CAD build for the part. Positions are in the model's coordinates, mm. A direction names the side the tool comes from. Coordinates: 2 decimals unless noted, no trailing zeros. Loops run counter-clockwise (first coordinate to the right, second up) from the corner with the lowest first, then second, coordinate; pieces in that order, holes last. Notation, with made-up numbers: (24.25, -16.75) -> (69.25, -16.75) arc R11 cw to (69.25, -4.75) -> close; hole circle Ø11 at (82.25, 87). An arc over 180 degrees is marked (long way). Write each question's results on one line, items separated by ' | '.
Autodesk Inventor part; units mm, degrees
ref_plane "YZ Plane" through (0, 0, 0) normal (1, 0, 0) x (0, 1, 0)
ref_plane "XZ Plane" through (0, 0, 0) normal (0, 1, 0) x (-1, 0, 0)
ref_plane "XY Plane" through (0, 0, 0) normal (0, 0, 1) x (1, 0, 0)
sketch "スケッチ1" plane through (0, 0, 0) normal (0, 1, 0) x (-1, 0, 0)
  line L0 (0, 0) -> (20, 0)
  line L1 (20, 0) -> (20, -40)
  line L2 (20, -40) -> (0, -40)
  line L3 (0, -40) -> (0, 0)
  circle A0 centre (0, -20) radius 13.6
  circle A1 centre (0, -20) radius 17.5
  line L4 (0, -6.4) -> (4, -6.4)
  line L5 (4, -6.4) -> (4, 3.6)
  line L6 (4, 3.6) -> (0, 3.6)
  line L7 (0, 3.6) -> (0, -6.4)
  line L8 (0, -33.6) -> (4, -33.6)
  line L9 (4, -33.6) -> (4, -43.6)
  line L10 (4, -43.6) -> (0, -43.6)
  line L11 (0, -43.6) -> (0, -33.6)
  point P0 (0, -6.4)
  point P1 (0, -33.6)
  point P2 (4, -37.0367)
  point P3 (4, -2.9633)
  dimension "d0" = 20
  dimension "d1" = 40
  dimension "d2" = 27.2
  dimension "d3" = 35
  dimension "d4" = 4
  dimension "d5" = 10
  dimension "d6" = 4
  dimension "d7" = 10
extrude "押し出し1" add sketch "スケッチ1" along normal blind 87 contours L7 L6 L5 L0 | L0 L5 A1 L3 | A1 L5 L4 L3 | A1 L9 L8 A0 L4 L5 | A1 L9 L2 L3 | L3 L8 L9 A1 | L2 L9 L10 L11
sketch "スケッチ2" plane through (-4, 0, -43.6) normal (-1, 0, 0) x (0, 0, 1)
  line L0 (0, 87) -> (6.5633, 87)
  line L1 (40.6367, 87) -> (47.2, 87)
  line L2 (40.6367, 0) -> (47.2, 0)
  line L3 (0, 0) -> (6.5633, 0)
  point P0 (43.6, 0)
  point P1 (3.2816, 13)
  point P2 (3.2816, 79)
  point P3 (43.9184, 79)
  point P4 (43.9184, 13)
  point P5 (3.2816, 87)
  point P6 (43.9184, 87)
  point P7 (43.9184, 0)
  point P8 (3.2816, 0)
  dimension "d10" = 0
  dimension "d11" = 8
  dimension "d12" = 0
  dimension "d13" = 8
  dimension "d14" = 0
  dimension "d15" = 0
  dimension "d16" = 13
  dimension "d17" = 13
hole "穴1" at (-4, 13, -40.3184) at (-4, 79, -40.3184) at (-4, 79, 0.3184) at (-4, 13, 0.3184) direction (1, 0, 0) diameter 3 end through all
fillet "フィレット1" radius 1 14 edges at (-4, 87, 0.3184) (-17.5, 87, -20) (-4, 87, -40.3184) (-2, 87, -43.6) (-2, 87, 3.6) (-4, 43.5, 3.6) (-4, 0, 0.3184) (-17.5, 0, -20) (-4, 0, -40.3184) (-2, 0, -43.6) (-2, 0, 3.6) (-4, 43.5, -43.6) (-4, 43.5, -37.0367) (-4, 43.5, -2.9633)
sketch "スケッチ3" plane through (0, 87, 0) normal (0, 1, 0) x (1, 0, 0)
  line L0 (0, -2.6) -> (-3, -2.6)
  line L1 (-3, 42.6) -> (0, 42.6)
  circle A0 centre (-1.5, 39.6) radius 0.5
  circle A1 centre (-1.5, 0.4) radius 0.5
  circle A2 centre (-15.1647, 20) radius 0.5
  arc A3 (-4.7297, 36.8487) -> (-4.7297, 3.1513) centre (0, 20) ccw
  point P0 (-17.5, 20)
  dimension "d28" = 3
  dimension "d29" = 3
  dimension "d30" = 1
  dimension "d31" = 1
  dimension "d32" = 1
  dimension "d33" = 0
extrude "押し出し2" add sketch "スケッチ3" along normal blind 2
sketch "スケッチ4" plane through (-1.5, 89, -39.6) normal (0, 1, 0) x (1, 0, 0)
  line L0 (-16.7138, 4.8708) -> (4.6687, 4.8708)
  line L1 (4.6687, 4.8708) -> (4.6687, -44.2225)
  line L2 (4.6687, -44.2225) -> (-16.7138, -44.2225)
  line L3 (-16.7138, -44.2225) -> (-16.7138, 4.8708)
  point P0 (1.5, -39.6)
extrude "押し出し3" add sketch "スケッチ4" along normal blind 1
sketch "スケッチ5" plane through (-4, 1, -37.8115) normal (-1, 0, 0) x (0, 0, 1)
  circle A0 centre (-2.5068, 12) radius 1.5
  circle A1 centre (-2.5068, 12) radius 2.5
  circle A2 centre (38.1299, 12) radius 1.5
  circle A3 centre (38.1299, 12) radius 2.5
  circle A4 centre (-2.5068, 78) radius 1.5
  circle A5 centre (-2.5068, 78) radius 2.5
  circle A6 centre (38.1299, 78) radius 1.5
  circle A7 centre (38.1299, 78) radius 2.5
  point P0 (37.8115, -1)
  dimension "d36" = 5
  dimension "d37" = 5
  dimension "d38" = 5
  dimension "d39" = 5
extrude "押し出し4" cut sketch "スケッチ5" against normal blind 2
properties part number "arm-2-2_3D プリント"
Q1. Cut at B-B on y = 13. Give the number of separate pieces and of enclosed holes in the cut face, and give its area (3 significant figures).
Results are:
separate pieces: 3 | enclosed holes: 0 | area: 208 mm^2
Q2. Wall check: L1, parallel to Z at x = -0.5, y = 79; L2, parallel to Z at x = -3.1, y = 79; L3, parallel to Y at x = -2, z = -35. Give the ranges that are in metal, low to high. Write a range as from..to.
Results are:
L1: -43.6..-41.82, -38.82..-33.59, -6.41..-1.18, 1.82..3.6 | L2: -43.59..-42.82, -37.82..-33.24, -6.76..-2.18, 2.82..3.59 | L3: 0..87, 89..90
Q3. Pull direction Z, two halves, no side cores. Call faces 5 (the flat face through (0, 43, -1)), 6 (the cylindrical face through (-3.01, 10.56, -0.22)), 7 (the cylindrical face through (-0.986, 77.735, 1.125)), 8 (the cylindrical face through (-17.497, 42.905, -19.682)): +Z half, -Z half, draft (parallel to the pull), parting line (faces both ways), or undercut.
Results are:
face 5: draft | face 6: undercut | face 7: undercut | face 8: parting line
Q4. Which spindle directions (+Z, -Z, +X, -X, +Y, -Y) get a long thin tool onto all of the face, cutting with end or side? Do faces 1 (the flat face through (-4, 43, 0)), 2 (the cylindrical face through (-3.01, 78.04, -38.01)), 3 (the cylindrical face through (-13.597, 42.891, -19.701)), 4 (the flat face through (-2, 43, 3.6)). Say none if no direction does.
Results are:
face 1: +Z, -X, -Y | face 2: -X | face 3: +X, -Y | face 4: +Z, +X, -X, -Y
Q5. Cut at D-D on x = 1.5. Write the cut outline in (y, z), and give its area (3 significant figures).
Results are:
outline: (89, -44.47) -> (90, -44.47) -> (90, 4.62) -> (89, 4.62) -> close | area: 49.1 mm^2
Q6. Drop flat-ended pins along their axis: pin 1 (6 mm diameter, centred on y = 29, z = -9, fed in from -X); pin 2 (1.5 mm diameter, centred on x = -1, y = 25, fed in from -Z); pin 3 (4 mm diameter, centred on x = -7, y = 16.5, fed in from -Z); pin 4 (1.8 mm diameter, centred on y = 13, z = 0.32, fed in from -X). Give the stop position or say it passes through.
Results are:
pin 1: x = -15.56 | pin 2: z = -43.6 | pin 3: z = -36.77 | pin 4: through
Q7. Cut at A-A on y = 40. Write the cut outline in (x, z).
Results are:
outline: (-4.73, -36.85) arc R1 cw to (-4, -37.81) -> (-4, -42.6) arc R1 ccw to (-3, -43.6) -> (0, -43.6) -> (0, -33.6) arc R13.6 cw to (0, -6.4) -> (0, 3.6) -> (-3, 3.6) arc R1 ccw to (-4, 2.6) -> (-4, -2.19) arc R1 cw to (-4.73, -3.15) arc R17.5 ccw to start
